from build123d import *

# Parameters (mm, degrees)
BOSS_EXTRUDE1_DEPTH        = 10
SKETCH2_W                  = 5.05
SKETCH2_H                  = 7.05
CUT_EXTRUDE6_DEPTH         = 10
CUT_EXTRUDE7_DEPTH         = 5
CHAMFER2_SIZE              = 5.196152423
CHAMFER2_SIZE_2            = 9
CHAMFER2_OF_MIRROR4_SIZE   = 5.196152423
CHAMFER2_OF_MIRROR4_SIZE_2 = 9
SKETCH5_R                  = 2
CUT_EXTRUDE5_DEPTH         = 6
CUT_EXTRUDE8_START         = -120
CUT_EXTRUDE8_DEPTH         = 24.374622763
SKETCH8_R                  = 144.95
CUT_EXTRUDE9_DEPTH         = 12
BOSS_EXTRUDE2_DEPTH        = 20


# Read off the part's stored shape, not the designer's step: Cut-Extrude8
with BuildPart() as part:
    # Sketch1 → Boss-Extrude1 (new, symmetric)
    with BuildSketch(Plane.XY):
        Polygon((0, 120), (0, 80), (-10, 80), (-87.75, 12), (-87.75, 0), (-102.75, 0), (-102.75, 24), (-20, 120), align=None)
    extrude(amount=BOSS_EXTRUDE1_DEPTH, both=True)

    # Sketch2 → Cut-Extrude6 (cut)
    with BuildSketch(Plane.XZ):
        with Locations((-100.225, 6.475)):
            Rectangle(SKETCH2_W, SKETCH2_H)
        with Locations((-90.275, 6.475)):
            Rectangle(SKETCH2_W, SKETCH2_H)
        with Locations((-90.275, -6.475)):
            Rectangle(SKETCH2_W, SKETCH2_H)
        with Locations((-100.225, -6.475)):
            Rectangle(SKETCH2_W, SKETCH2_H)
    extrude(amount=-CUT_EXTRUDE6_DEPTH, mode=Mode.SUBTRACT)

    # Sketch6 → Cut-Extrude7 (cut)
    with BuildSketch(Plane.XY.offset(10)):
        Polygon((-98.494242528, 28.937192959), (-85.75, 13.749196141), (-13, 77.376205788), (-25.986145629, 113.055347669), align=None)
    cut_extrude7 = extrude(amount=-CUT_EXTRUDE7_DEPTH, mode=Mode.SUBTRACT)

    # Chamfer2
    # the kernel refuses this chamfer: 9, 5.196152423 mm, written as the material it adds along each edge
    with BuildSketch(Plane(origin=(-5.036481035, 55.496617251, 5), x_dir=(0.05440243528858507, 0.019800867116638043, 0.9983227437537925), z_dir=(-0.342020143325666, 0.9396926207859094, 0))) as chamfer2_piece_1_section:
        Polygon((CHAMFER2_SIZE * 0.998322743697, -CHAMFER2_SIZE * 0.0578938623994), (-CHAMFER2_SIZE_2 * 0.0578938624027, -CHAMFER2_SIZE_2 * 0.998322743754), (0, 0), align=None)
    chamfer2_piece_1 = extrude(amount=84.536493315, mode=Mode.PRIVATE)
    chamfer2_piece_1 = split(chamfer2_piece_1, bisect_by=Plane(origin=(-21.83844233, 92.842389445, 10), z_dir=(0, 0, -1)), keep=Keep.TOP, mode=Mode.PRIVATE)
    chamfer2_piece_1 = split(chamfer2_piece_1, bisect_by=Plane(origin=(-34.214088998, 103.509939047, 6.650101228), z_dir=(0.7574435982041207, -0.6529006015769894, 0)), keep=Keep.TOP, mode=Mode.PRIVATE)
    chamfer2_piece_1 = split(chamfer2_piece_1, bisect_by=Plane(origin=(-10.343648825, 79.699445401, 6.650101228), z_dir=(-0.6583332390976693, 0.7527266079388791, 0)), keep=Keep.TOP, mode=Mode.PRIVATE)
    add(chamfer2_piece_1)
    with BuildSketch(Plane(origin=(-113.460762542, 46.773596955, 5), x_dir=(-0.04434927158426045, -0.03721345742933334, 0.9983227437537927), z_dir=(0.642787609686533, -0.7660444431189835, 0))) as chamfer2_piece_2_section:
        Polygon((CHAMFER2_SIZE * 0.998322743697, -CHAMFER2_SIZE * 0.0578938623994), (-CHAMFER2_SIZE_2 * 0.0578938624027, -CHAMFER2_SIZE_2 * 0.998322743754), (0, 0), align=None)
    chamfer2_piece_2 = extrude(amount=66.394065339, mode=Mode.PRIVATE)
    chamfer2_piece_2 = split(chamfer2_piece_2, bisect_by=Plane(origin=(-97.520772346, 30.066536009, 6.631431033), z_dir=(0.7574435982041207, -0.6529006015769894, 0)), keep=Keep.TOP, mode=Mode.PRIVATE)
    chamfer2_piece_2 = split(chamfer2_piece_2, bisect_by=Plane(origin=(-83.277010041, 15.912068389, 6.631431033), z_dir=(-0.6583332390976693, 0.7527266079388791, 0)), keep=Keep.TOP, mode=Mode.PRIVATE)
    chamfer2_piece_2 = split(chamfer2_piece_2, bisect_by=Plane(origin=(-89.945880011, 23.537136627, 10), z_dir=(0, 0, -1)), keep=Keep.TOP, mode=Mode.PRIVATE)
    add(chamfer2_piece_2)

    # Mirror4: Cut-Extrude7 across plane
    add(cut_extrude7.mirror(Plane.XY), mode=Mode.SUBTRACT)

    # Chamfer2 of Mirror4
    # the kernel refuses this chamfer: 9, 5.196152423 mm, written as the material it adds along each edge
    with BuildSketch(Plane(origin=(-5.036481035, 55.496617251, -5), x_dir=(0.05440243528858507, 0.019800867116638043, -0.9983227437537925), z_dir=(-0.342020143325666, 0.9396926207859094, 0))) as chamfer2_of_mirror4_piece_1_section:
        Polygon((CHAMFER2_OF_MIRROR4_SIZE * 0.998322743697, CHAMFER2_OF_MIRROR4_SIZE * 0.0578938623994), (-CHAMFER2_OF_MIRROR4_SIZE_2 * 0.0578938624027, CHAMFER2_OF_MIRROR4_SIZE_2 * 0.998322743754), (0, 0), align=None)
    chamfer2_of_mirror4_piece_1 = extrude(amount=84.536493315, mode=Mode.PRIVATE)
    chamfer2_of_mirror4_piece_1 = split(chamfer2_of_mirror4_piece_1, bisect_by=Plane(origin=(-34.214088998, 103.509939047, -6.650101228), z_dir=(0.7574435982040639, -0.6529006015770552, 0)), keep=Keep.TOP, mode=Mode.PRIVATE)
    chamfer2_of_mirror4_piece_1 = split(chamfer2_of_mirror4_piece_1, bisect_by=Plane(origin=(-10.343648825, 79.699445401, -6.650101228), z_dir=(-0.6583332390977968, 0.7527266079387677, 0)), keep=Keep.TOP, mode=Mode.PRIVATE)
    chamfer2_of_mirror4_piece_1 = split(chamfer2_of_mirror4_piece_1, bisect_by=Plane(origin=(-21.83844233, 92.842389445, -10), z_dir=(0, 0, 1)), keep=Keep.TOP, mode=Mode.PRIVATE)
    add(chamfer2_of_mirror4_piece_1)
    with BuildSketch(Plane(origin=(-113.460762542, 46.773596955, -5), x_dir=(0.7659013618145366, 0.6426675502167433, 0.019326765612700778), z_dir=(0.642787609686533, -0.7660444431189835, 0))) as chamfer2_of_mirror4_piece_2_section:
        Polygon((CHAMFER2_OF_MIRROR4_SIZE_2 * 0.999813220622, -CHAMFER2_OF_MIRROR4_SIZE_2 * 0.0193267656127), (-CHAMFER2_OF_MIRROR4_SIZE * 0.0193267656116, -CHAMFER2_OF_MIRROR4_SIZE * 0.999813220566), (0, 0), align=None)
    chamfer2_of_mirror4_piece_2 = extrude(amount=66.394065339, mode=Mode.PRIVATE)
    chamfer2_of_mirror4_piece_2 = split(chamfer2_of_mirror4_piece_2, bisect_by=Plane(origin=(-97.520772346, 30.066536009, -6.631431033), z_dir=(0.7574435982040639, -0.6529006015770552, 0)), keep=Keep.TOP, mode=Mode.PRIVATE)
    chamfer2_of_mirror4_piece_2 = split(chamfer2_of_mirror4_piece_2, bisect_by=Plane(origin=(-83.277010041, 15.912068389, -6.631431033), z_dir=(-0.6583332390977968, 0.7527266079387677, 0)), keep=Keep.TOP, mode=Mode.PRIVATE)
    chamfer2_of_mirror4_piece_2 = split(chamfer2_of_mirror4_piece_2, bisect_by=Plane(origin=(-89.945880011, 23.537136627, -10), z_dir=(0, 0, 1)), keep=Keep.TOP, mode=Mode.PRIVATE)
    add(chamfer2_of_mirror4_piece_2)

    # Sketch5 → Cut-Extrude5 (cut)
    with BuildSketch(Plane(origin=(0, 0, 0), x_dir=(0, 0, -1), z_dir=(1, 0, 0))):
        with Locations((-5, 112.75)):
            Circle(SKETCH5_R)
        with Locations((-5, 87.25)):
            Circle(SKETCH5_R)
        with Locations(Location((5, 87.25, 0), (0, 0, 180))):
            Circle(SKETCH5_R)
        with Locations(Location((5, 112.75, 0), (0, 0, 180))):
            Circle(SKETCH5_R)
    extrude(amount=-CUT_EXTRUDE5_DEPTH, mode=Mode.SUBTRACT)

    # Cut-Extrude8 outline → Cut-Extrude8 (cut)
    with BuildSketch(Plane(origin=(0, 120, 0), x_dir=(1, 0, 0), z_dir=(0, 1, 0)).offset(CUT_EXTRUDE8_START)):
        with BuildLine():
            Line((-102.75, 7.56e-07), (-102.75, -10))
            Line((-102.75, -10), (-102.427082983, -10))
            ThreePointArc((-102.427082983, -10), (-102.669249724, -5.002605828), (-102.75, 7.56e-07))
        make_face()
        with BuildLine():
            Line((-102.427082983, 10), (-102.75, 10))
            Line((-102.75, 10), (-102.75, 7.56e-07))
            ThreePointArc((-102.75, 7.56e-07), (-102.669249699, 5.002606583), (-102.427082983, 10))
        make_face()
    extrude(amount=CUT_EXTRUDE8_DEPTH, mode=Mode.SUBTRACT)

    # Sketch8 → Cut-Extrude9 (cut)
    with BuildSketch(Plane.XZ):
        with Locations((56.25, 0)):
            Circle(SKETCH8_R)
    extrude(amount=-CUT_EXTRUDE9_DEPTH, mode=Mode.SUBTRACT)

    # Sketch10 → Boss-Extrude2 (add)
    with BuildSketch(Plane(origin=(0, 0, -10), x_dir=(-1, 0, 0), z_dir=(0, 0, -1))):
        Polygon((87.75, 12), (88.771540348, 10.230640215), (90.560927794, 10.230640215), (90.560927794, 12), align=None)
    extrude(amount=-BOSS_EXTRUDE2_DEPTH)


solid = part.part
Geometry: final body of the model. Coordinates: model frame, mm. A direction names the side the tool comes from. Round coordinates to 2 decimals unless told otherwise and drop trailing zeros. Loops run counter-clockwise (first coordinate to the right, second up) from the corner with the lowest first, then second, coordinate; pieces in that order, holes last. Notation, with made-up numbers: M -39.75,22 L -9.75,22 A29 cw -9.75,46 Z; hole C -24,32 d1. An arc over 180 degrees is marked long. One line per question, with ' | ' between items.
(1) Pull-direction query (Y, two-part tool) for faces 1 (the cylindrical face through (-2.958, 111.064, -3.925)), 2 (the flat face through (-57, 63, -5)), 3 (the flat face through (-23.097, 91.641, -7.535)), 4 (the flat face through (-61.95, 71.33, 0.14)); classes: +Y half, -Y half, draft (parallel to the pull), parting line (faces both ways), or undercut.
Check result:
face 1: undercut | face 2: draft | face 3: -Y half | face 4: +Y half
(2) Material intervals for line 1 along Z through (x, y) = (-1, 87); line 2 along Y through (x, z) = (-4.3, 5); line 3 along Z through (x, y) = (-1, 112), sorted ascending. Write a range as from..to.
Check result:
line 1: z = -10..-6.98, -3.02..3.02, 6.98..10 | line 2: y = 80..85.25, 89.25..110.75, 114.75..120 | line 3: z = -10..-6.85, -3.15..3.15, 6.85..10
(3) Contact query for flat-ended pins moving along their axis: P1, Ø10, axis at x = -25.5, z = 4.5, coming from the -Y side; P2, Ø2, axis at y = 3.5, z = -7, coming from the -X side; P3, Ø12, axis at y = 38.5, z = -6, coming from the +X side. Output: stop coordinate, or through.
Check result:
P1: stops at y = 62.07 | P2: stops at x = -97.7 | P3: stops at x = -50.69
(4) Cut plane C-C on x = -60. Return the cut outline in (y, z).
Check result:
outline: M 36.27,-5 L 73.6,-5 L 73.6,5 L 36.27,5 Z
(5) Access query for faces 5 (the flat face through (-97.7, 5, 6)), 6 (the flat face through (-6, 87, 5)), 7 (the flat face through (-91, 10, 7)). Directions: +Z, -Z, +X, -X, +Y, -Y. A direction counts if a zero-diameter tool reaches every point of the face in a straight line with its end or side. Return the directions, or none.
Check result:
face 5: +Z, -X, -Y | face 6: +X | face 7: +Z, +X, -Y
(6) Cut plane A-A on y = 95.5. Return the cut outline in (x, z), plus the area to 3 significant figures.
Check result:
outline: M -41.12,-5 L -29.17,-5 L -19.96,-10 L 0,-10 L 0,10 L -19.96,10 L -29.17,5 L -41.12,5 Z | area: 657 mm2
(7) Cut plane D-D on x = -39. Return the cut outline in (y, z), plus the area to 3 significant figures.
Check result:
outline: M 54.64,-5 L 97.96,-5 L 97.96,5 L 54.64,5 Z | area: 433 mm2
(8) Cut plane B-B on x = -16. Return the cut outline in (y, z).
Check result:
outline: M 74.75,-8.05 L 84.63,-10 L 120,-10 L 120,10 L 84.63,10 L 74.75,8.05 Z
